Could you check a few things on this model? Use its own coordinates, in mm. A direction names the side the tool comes from. Give positions to 0.01 mm unless a question says otherwise; leave off trailing zeros. Write each loop counter-clockwise with the first axis right and the second up, starting at its lowest first coordinate (ties: lowest second). Pieces come first, ordered by that corner, then holes. Notation, with made-up numbers: M 86.5,60 L 110.5,60 A25 ccw 110.5,77 Z; hole C 76.5,50.5 d2. An arc over 180 degrees is marked long. Use one line per item in the form item = value.
from build123d import *

# Parameters (mm, degrees)
F1_DEPTH = 508
F3_DEPTH = 254
F5_DEPTH = 254


with BuildPart() as f1:
    # F0 (on Front) → F1 (new body)
    with BuildSketch(Plane.XZ):
        Polygon((-22.912122, 26.238084), (-50.258853, 33.43459), (-50.258853, -33.629075), (35.476834, -53.215235), (54.221553, 28.837158), (28.085828, 28.837158), (15.890658, 49.519747), (-22.912122, 46.932891), align=None)
    extrude(amount=F1_DEPTH)

    # F2 (on face) → F3 (join)
    with BuildSketch(Plane(origin=(0, 0, 0), x_dir=(-1, 0, 0), z_dir=(0, 1, 0))):
        Polygon((28.587002, 10.809334), (-5.875511, 11.1418), (-6.94721, 10.140639), (-24.068851, 12.258933), (-25.929179, -8.414216), (0, -22.702822), (16.708504, -22.702822), (31.25754, -10.755406), align=None)
    extrude(amount=-F3_DEPTH)

    # F4 (on Front) → F5 (join)
    with BuildSketch(Plane.XZ):
        Polygon((21.636747, -16.150855), (21.636747, 12.28594), (25.461577, 15.112989), (31.614564, 26.254892), (7.335201, 23.926727), (-1.644839, 34.56974), (-20.935295, 13.616316), (-33.906464, -2.84709), (-24.760127, -19.1442), (-13.618225, -9.997867), (-3.474105, -22.470139), align=None)
    extrude(amount=-F5_DEPTH)


solid = f1.part
1) For faces 5 (the flat face through (19.645, 125.222, 25.107)), 6 (the flat face through (-29.4, 125.22, -10.88)), 7 (the flat face through (-11.155, 125.222, 24.24)), 8 (the flat face through (-22.912, -250, 37)), which set-ups out of +Z, -Z, +X, -X, +Y, -Y let a thin tool reach every point of the face, with its end or its side?
Checked values:
face_5 = +Z, +Y
face_6 = -Z, -X, +Y
face_7 = +Z, -X, +Y
face_8 = +Z, +Y, -Y
2) If I drill on L1, parallel to Y at x = 48, z = 6; L2, parallel to X at y = -104.5, z = -2.5; L3, parallel to Z at x = 12.5, y = -220, over which ranges is the centre line in solid material (lowest first)?
Checked values:
L1 = -508 to 0
L2 = -50.26 to 47.06
L3 = -47.97 to 49.29
3) I want a section at C-C, the plane y = 166.5. Please give me the cut outline in (x, z), plus the area to 3 significant figures.
Checked values:
outline = M -33.91,-2.85 L -24.76,-19.14 L -13.62,-10 L -3.47,-22.47 L 21.64,-16.15 L 21.64,12.29 L 25.46,15.11 L 31.61,26.25 L 7.34,23.93 L -1.64,34.57 L -20.94,13.62 Z
area = 2,140 mm2
4) For pin 1 Ø1.5 at (y, z) = (-269.5, -33.5) entering from +X; pin 2 Ø1.5 at (y, z) = (-293.5, 27) entering from +X; pin 3 Ø1.5 at (y, z) = (100, -19) entering from -X, each with a flat end and sliding along its axis, tell me the tip position at first contact or that it passes through.
Checked values:
pin_1 = 40.15
pin_2 = 53.97
pin_3 = -25.26
5) I want a section at B-B, the plane z = -43. Please give me the cut outline in (x, y).
Checked values:
outline = M -9.24,-508 L 37.81,-508 L 37.81,0 L -9.24,0 Z
6) I want a section at A-A, the plane y = -225. Please give me the cut outline in (x, z), plus the area to 3 significant figures.
Checked values:
outline = M -50.26,-33.63 L 35.48,-53.22 L 54.22,28.84 L 28.09,28.84 L 15.89,49.52 L -22.91,46.93 L -22.91,26.24 L -50.26,33.43 Z
area = 7,870 mm2
7) Thinking about a two-plate mould opening in X: for faces 1 (the flat face through (-36.394, -250.444, 29.786)), 2 (the flat face through (-8.617, 125.222, -16.147)), 3 (the flat face through (-7.991, -250.444, -43.285)), 4 (the flat face through (21.637, 125, -2)), which applies, released by +X, released by -X, zero draft, split by the parting line, or undercut?
Checked values:
face_1 = undercut
face_2 = undercut
face_3 = released by -X
face_4 = released by +X
